Autodesk Inventor part; units mm, degrees
ref_plane "YZ Plane" through (0, 0, 0) normal (1, 0, 0) x (0, 1, 0)
ref_plane "XZ Plane" through (0, 0, 0) normal (0, 1, 0) x (-1, 0, 0)
ref_plane "XY Plane" through (0, 0, 0) normal (0, 0, 1) x (1, 0, 0)
sketch "Boceto1" plane through (0, 0, 0) normal (0, 1, 0) x (-1, 0, 0)
  line L0 (0, 0) -> (0, -17.6)
  line L1 (0, -17.6) -> (7.5, -17.6)
  line L2 (7.5, -17.6) -> (7.5, 0)
  line L3 (7.5, 0) -> (0, 0)
  dimension "d0" = 17.6
  dimension "d1" = 7.5
extrude "Extrusión1" add sketch "Boceto1" along normal blind 3.3
sketch "Boceto2" plane through (0, 3.3, 0) normal (0, 1, 0) x (1, 0, 0)
  line L0 (0, 0) -> (0, 17.6)
  line L1 (0, 17.6) -> (-7.5, 17.6)
  line L2 (-7.5, 17.6) -> (-7.5, 0)
  line L3 (-7.5, 0) -> (0, 0)
  line L4 (-7, 0.5) -> (-7, 17.1)
  line L5 (-7, 17.1) -> (-0.5, 17.1)
  line L6 (-0.5, 17.1) -> (-0.5, 0.5)
  line L7 (-0.5, 0.5) -> (-7, 0.5)
  dimension "d4" = 0.5
extrude "Extrusión2" cut sketch "Boceto2" against normal blind 2.8 contours L4 L5 L6 L7
sketch "Boceto3" plane through (0, 3.3, 0) normal (0, 1, 0) x (1, 0, 0)
  line L0 (-0.5, 17.1) -> (-0.5, 0.5)
  line L1 (-0.5, 0.5) -> (0, 0.5)
  line L2 (0, 0.5) -> (0, 17.1)
  line L3 (0, 0) -> (0, 17.6)
  line L4 (-0.5, 17.1) -> (-0.5, 0.5)
  line L5 (-0.5, 17.1) -> (-0.5, 0.5)
  line L6 (-0.5, 0.5) -> (-0.5, 17.1)
  line L7 (-0.5, 17.1) -> (0, 17.1)
extrude "Extrusión3" cut sketch "Boceto3" against normal blind 0.5
sketch "Boceto4" plane through (0, 0, 0) normal (1, 0, 0) x (0, 0, -1)
  line L0 (0.5, 2.8) -> (0.5, 3.3)
  line L1 (0, 3.3) -> (0.5, 3.3)
  line L2 (0, 0) -> (0, 3.3)
  line L3 (0, 0) -> (17.6, 0)
  line L4 (17.6, 0) -> (17.6, 3.3)
  line L5 (17.1, 3.3) -> (17.6, 3.3)
  line L6 (17.1, 3.3) -> (17.1, 2.8)
  line L7 (17.1, 2.8) -> (0.5, 2.8)
  line L8 (0.5, 3.3) -> (0.5, 0.5)
  line L9 (0.5, 2.8) -> (0.5, 3.3)
  line L10 (0.5, 3.3) -> (0.5, 3.05)
  line L11 (0.5, 2.8) -> (0.25, 3.05)
  line L12 (0.5, 3.3) -> (0.25, 3.05)
  line L13 (17.1, 3.3) -> (17.1, 2.8)
  line L14 (17.1, 3.3) -> (17.6, 3.3)
  line L15 (17.1, 3.3) -> (17.35, 3.05)
  line L16 (17.35, 3.05) -> (17.1, 2.8)
extrude "Extrusión4" cut sketch "Boceto4" against normal blind 7 contours L11 L12 L0 | L6 L15 L16
sketch "Boceto5" plane through (0, 0, 0) normal (1, 0, 0) x (0, 0, -1)
  line L0 (0.5, 2.8) -> (17.1, 2.8)
  circle A0 centre (8.8, 2.8) radius 0.9
  line L1 (7.9, 2.8) -> (9.7, 2.8)
  point P0 (0, 0)
  dimension "d11" = 1.8
extrude "Extrusión5" cut sketch "Boceto5" against normal blind 5 contours L0 A0 picked at (8.728, 2.3801)
Here's how the part is built. I have some questions about the finished solid (model axes, mm). A direction names the side the tool comes from. Coordinates: 2 decimals unless noted, no trailing zeros. Write each loop counter-clockwise with the first axis right and the second up, starting at its lowest first coordinate (ties: lowest second). Pieces come first, ordered by that corner, then holes. Notation, with made-up numbers: (47, 34.25) - (59, 34.25) arc R5 ccw to (59, 41.25) - close; hole circle Ø5 at (45, 22.5). An arc over 180 degrees is marked (long way). One line per item, written item: value.
1) I need wall thicknesses on line 1 along Z through (x, y) = (-5.25, 1.2); line 2 along X through (y, z) = (1.1, -4); line 3 along Y through (x, z) = (-3, -14.5). Which ranges of each line are inside material? Lowest first, please.
Model answer:
line 1: z = -17.6 to -17.1, -0.5 to 0
line 2: x = -7.5 to -7, -0.5 to 0
line 3: y = 0 to 0.5
2) Suppose I cut it at B-B on x = -2. Write out the boundary of the cut face in (y, z), and give its area (3 significant figures).
Model answer:
outline: (0, -17.6) - (3.3, -17.6) - (3.3, -17.1) - (3.05, -17.35) - (2.8, -17.1) - (0.5, -17.1) - (0.5, -0.5) - (2.8, -0.5) - (3.05, -0.25) - (3.3, -0.5) - (3.3, 0) - (0, 0) - close
area: 11.5 mm²
3) I'm going to push flat-ended pins straight in: P1, Ø0.6, axis at x = 0, z = -13, coming from the +Y side; P2, Ø2, axis at x = -2.5, z = -12.5, coming from the +Y side. Where does each tip first touch, or does it pass through?
Model answer:
P1: stops at y = 2.8
P2: stops at y = 0.5
4) On a 3-axis mill with a long thin cutter (end or side, diameter ignored), from which of +Z, -Z, +X, -X, +Y, -Y can I reach the whole of each face in a straight line? I mean faces 1 (the flat face through (-4, 0, -9)), 2 (the flat face through (-4, 2, -0.5)), 3 (the cylindrical face through (-0.2, 1.9, -8.8)). Say none if no direction works.
Model answer:
face 1: +Z, -Z, +X, -X, -Y
face 2: +Y
face 3: +X, +Y
5) Suppose I cut it at A-A on z = -8.8. Write out the boundary of the cut face in (x, y), and give its area (3 significant figures).
Model answer:
outline: (-7.5, 0) - (0, 0) - (0, 1.9) - (-0.5, 1.9) - (-0.5, 0.5) - (-7, 0.5) - (-7, 3.3) - (-7.5, 3.3) - close
area: 5.85 mm²
6) We'd pull the mould along Z, two halves only. Please class faces 4 (the flat face through (-7.3, 3.3, -8.8)), 5 (the flat face through (-4, 2, 0)), 6 (the flat face through (-0.5, 1.7, -8.9)): pulls with the +Z half, pulls with the -Z half, needs draft (parallel to the pull), parting line crosses it, or undercut.
Model answer:
face 4: needs draft
face 5: pulls with the +Z half
face 6: undercut
